Verification items for the finished model (mm, model axes). A direction names the side the tool comes from. Coordinates: 2 decimals unless noted, no trailing zeros. Loops run counter-clockwise (first coordinate to the right, second up) from the corner with the lowest first, then second, coordinate; pieces in that order, holes last.
Q1. Sectioned sample at B-B (y = 87.5). Enter the section's corners in (x, z) (1 decimal).
Q2. Sectioned sample at A-A (x = -12.7). Enter the section's corners in (y, z).
Q3. Mould release check, pull along X, two halves, no side actions. Record for faces 5 (the face through (9.194, 209.461, 12.878)), 6 (the face through (-49.894, 113.055, -8.259)), 7 (the face through (-12, 63.5, 0)): +X half, -X half, draft (parallel to the pull), parting line (faces both ways), or undercut.
Q4. Sectioned sample at C-C (z = 48). Enter the section's corners in (x, y).
Q5. Go/stop test with flat-tipped pins: P1, Ø14, axis at x = -16.5, y = 210.5, coming from the +Z side; P2, Ø6, axis at y = 165.5, z = -14, coming from the +X side; P3, Ø8, axis at x = 16, y = 140, coming from the +Z side. Record where each tip stops, or that it passes through.
Q6. Access from +Z, -Z, +X, -X, +Y, -Y to the whole of each face (thin tool, end or side, straight path). Record for faces 1 (the face through (-13, 209, 25.4)), 2 (the face through (-34.594, 209.461, -12.878)), 3 (the face through (-38, 203.2, -9)), 4 (the face through (9.4, 209.46, -12.52)).
Q7. Sectioned sample at D-D (y = 31). Enter the section's corners in (x, z).
Q8. Material ranges on probe 1 along Z at (x, y) = (-12, 141); probe 2 along X at (y, z) = (142, 0); probe 3 along Y at (x, z) = (4, 30.5), recorded low to high.
```python
from build123d import *

# Parameters (mm, degrees)
SKETCH1_W           = 127
SKETCH1_H           = 127
BOSS_EXTRUDE1_DEPTH = 25.4
SKETCH2_R           = 38.1
BOSS_EXTRUDE2_DEPTH = 177.8
BOSS_EXTRUDE3_DEPTH = 12.7
SKETCH4_R           = 17.4625
CUT_EXTRUDE1_DEPTH  = 152.4


with BuildPart() as part:
    # Sketch1 → Boss-Extrude1 (new body)
    with BuildSketch(Plane(origin=(0, 0, 0), x_dir=(1, 0, 0), z_dir=(0, 1, 0))):
        Rectangle(SKETCH1_W, SKETCH1_H)
    extrude(amount=BOSS_EXTRUDE1_DEPTH)

    # Sketch2 → Boss-Extrude2 (add)
    with BuildSketch(Plane(origin=(0, 25.4, 0), x_dir=(1, 0, 0), z_dir=(0, 1, 0))):
        with Locations(Location((-12.7, 0, 0), (0, 0, 270))):  # turned: the seam where the file's is
            Circle(SKETCH2_R)
    extrude(amount=BOSS_EXTRUDE2_DEPTH)

    # Sketch3 → Boss-Extrude3 (add)
    with BuildSketch(Plane(origin=(0, 203.2, 0), x_dir=(1, 0, 0), z_dir=(0, 1, 0))):
        Polygon((16.629393675, 0), (1.964696837, 25.4), (-27.364696837, 25.4), (-42.029393675, 0), (-27.364696837, -25.4), (1.964696837, -25.4), align=None)
    extrude(amount=BOSS_EXTRUDE3_DEPTH)

    # Sketch4 → Cut-Extrude1 (cut)
    with BuildSketch(Plane(origin=(0, 215.9, 0), x_dir=(1, 0, 0), z_dir=(0, 1, 0))):
        with Locations(Location((-12.7, 0, 0), (0, 0, 270))):  # turned: the seam where the file's is
            Circle(SKETCH4_R)
    extrude(amount=-CUT_EXTRUDE1_DEPTH, mode=Mode.SUBTRACT)


solid = part.part
```
Geometry check:
1. outline: circle Ø76.2 at (-12.7, 0); hole circle Ø34.9 at (-12.7, 0)
2. outline: (0, -63.5) - (25.4, -63.5) - (25.4, -38.1) - (203.2, -38.1) - (203.2, -25.4) - (215.9, -25.4) - (215.9, -17.46) - (63.5, -17.46) - (63.5, 17.46) - (215.9, 17.46) - (215.9, 25.4) - (203.2, 25.4) - (203.2, 38.1) - (25.4, 38.1) - (25.4, 63.5) - (0, 63.5) - close
3. face 5: +X half
3. face 6: parting line
3. face 7: undercut
4. outline: (-63.5, 0) - (63.5, 0) - (63.5, 25.4) - (-63.5, 25.4) - close
5. P1: stops at z = 25.4
5. P2: stops at x = 23.78
5. P3: stops at z = 29.01
6. face 1: +Z, +X, -X, +Y
6. face 2: -Z, -X, +Y
6. face 3: +Y
6. face 4: -Z, +X, +Y
7. outline: circle Ø76.2 at (-12.7, 0)
8. probe 1: z = -38.09 to -17.45, 17.45 to 38.09
8. probe 2: x = -50.8 to -30.16, 4.76 to 25.4
8. probe 3: y = 0 to 203.2
